For this review, take the finished solid that the model builds, in its own axes (mm). Face numbers are marked on the shaded views. Give positions to 0.01 mm unless a question says otherwise; leave off trailing zeros. Write each loop counter-clockwise with the first axis right and the second up, starting at its lowest first coordinate (ties: lowest second). Pieces come first, ordered by that corner, then holes.
1) We need section D-D on x = -21.5. Give the boundary of the cut face in (y, z), and give its area (3 significant figures).
2) For P1, Ø2, axis at x = -15, z = 26.5, coming from the +Y side; P2, Ø12, axis at x = -3, z = 56.5, coming from the -Y side; P3, Ø3.5, axis at y = -11.5, z = 37.5, coming from the +X side, all flat-tipped, find the tip position at first contact; note any pin that passes through.
3) We need section A-A on y = 0. Give the boundary of the cut face in (x, z), and give its area (3 significant figures).
4) We need section C-C on z = 46. Give the boundary of the cut face in (x, y).
5) Wall thickness on line 1 along Y through (x, z) = (10.75, 0.95); line 2 along Y through (x, z) = (3.5, 58); line 3 along Y through (x, z) = (-13.55, 21): over which ranges is each line inside the solid? List them lowest first.
6) We need section B-B on x = 0. Give the boundary of the cut face in (y, z), and give its area (3 significant figures).
7) Draft analysis for pull direction Y (two halves, no side actions). For the marked faces 1, 2 and 3, state which applies: pulls with the +Y half, pulls with the -Y half, needs draft (parallel to the pull), parting line crosses it, or undercut.
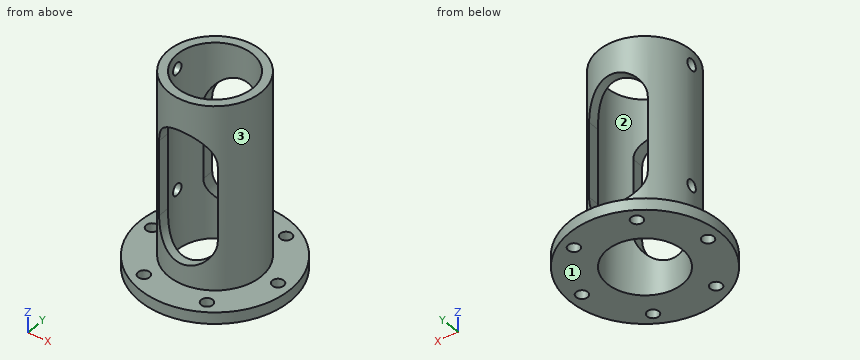
from build123d import *

# Parameters (mm, degrees)
SKETCH1_R           = 26
SKETCH1_R_2         = 13
SKETCH1_R_3         = 2
BOSS_EXTRUDE1_DEPTH = 4
SKETCH2_R           = 16
SKETCH2_R_2         = 13
BOSS_EXTRUDE2_DEPTH = 64
CUT_EXTRUDE1_DEPTH  = 32
SKETCH4_R           = 2
CUT_EXTRUDE2_DEPTH  = 64


with BuildPart() as part:
    # Sketch1 → Boss-Extrude1 (new body)
    with BuildSketch(Plane.XY):
        Circle(SKETCH1_R)
        Circle(SKETCH1_R_2, mode=Mode.SUBTRACT)
        with Locations((-21.5, 0)):
            Circle(SKETCH1_R_3, mode=Mode.SUBTRACT)
        with Locations((-10.75, 18.619546181)):
            Circle(SKETCH1_R_3, mode=Mode.SUBTRACT)
        with Locations((10.75, 18.619546181)):
            Circle(SKETCH1_R_3, mode=Mode.SUBTRACT)
        with Locations((21.5, 0)):
            Circle(SKETCH1_R_3, mode=Mode.SUBTRACT)
        with Locations((10.75, -18.619546181)):
            Circle(SKETCH1_R_3, mode=Mode.SUBTRACT)
        with Locations((-10.75, -18.619546181)):
            Circle(SKETCH1_R_3, mode=Mode.SUBTRACT)
    extrude(amount=BOSS_EXTRUDE1_DEPTH)

    # Sketch2 → Boss-Extrude2 (add)
    with BuildSketch(Plane.XY.offset(4)):
        Circle(SKETCH2_R)
        Circle(SKETCH2_R_2, mode=Mode.SUBTRACT)
    extrude(amount=BOSS_EXTRUDE2_DEPTH)

    # Sketch3 → Cut-Extrude1 (cut, symmetric)
    with BuildSketch(Plane(origin=(0, 0, 0), x_dir=(1, 0, 0), z_dir=(0, 1, 0))):
        with BuildLine():
            Line((10, -21), (10, -47))
            ThreePointArc((10, -47), (0, -57), (-10, -47))
            Line((-10, -47), (-10, -21))
            ThreePointArc((-10, -21), (0, -11), (10, -21))
        make_face()
    extrude(amount=CUT_EXTRUDE1_DEPTH, both=True, mode=Mode.SUBTRACT)

    # Sketch4 → Cut-Extrude2 (cut)
    with BuildSketch(Plane(origin=(0, 0, 0), x_dir=(0, 0, -1), z_dir=(1, 0, 0))):
        with Locations(Location((-21, 0, 0), (0, 0, 180))):
            Circle(SKETCH4_R)
        with Locations(Location((-63, 0, 0), (0, 0, 180))):
            Circle(SKETCH4_R)
    extrude(amount=-CUT_EXTRUDE2_DEPTH, mode=Mode.SUBTRACT)


solid = part.part
Results list:
1. outline: (-14.62, 0) - (-2, 0) - (-2, 4) - (-14.62, 4) - close; (2, 0) - (14.62, 0) - (14.62, 4) - (2, 4) - close
1. area: 101 mm2
2. P1: stops at y = 7.75
2. P2: stops at y = -16
2. P3: stops at x = 12.69
3. outline: (-26, 0) - (-23.5, 0) - (-23.5, 4) - (-26, 4) - close; (-19.5, 0) - (-13, 0) - (-13, 19) - (-16, 19) - (-16, 4) - (-19.5, 4) - close; (-16, 23) - (-13, 23) - (-13, 61) - (-16, 61) - close; (-16, 65) - (-13, 65) - (-13, 68) - (-16, 68) - close; (13, 0) - (19.5, 0) - (19.5, 4) - (16, 4) - (16, 68) - (13, 68) - close; (23.5, 0) - (26, 0) - (26, 4) - (23.5, 4) - close
3. area: 432 mm2
4. outline: (-10, -12.49) - (-10, -8.31) arc R13 cw to (-10, 8.31) - (-10, 12.49) arc R16 ccw to start; (10, -12.49) arc R16 ccw to (10, 12.49) - (10, 8.31) arc R13 cw to (10, -8.31) - close
5. line 1: y = -23.67 to -20.62, -16.62 to -7.31, 7.31 to 16.62, 20.62 to 23.67
5. line 2: y = -15.61 to -12.52, 12.52 to 15.61
5. line 3: y = -8.51 to -2, 2 to 8.51
6. outline: (-26, 0) - (-13, 0) - (-13, 11) - (-16, 11) - (-16, 4) - (-26, 4) - close; (-16, 57) - (-13, 57) - (-13, 68) - (-16, 68) - close; (13, 0) - (26, 0) - (26, 4) - (16, 4) - (16, 11) - (13, 11) - close; (13, 57) - (16, 57) - (16, 68) - (13, 68) - close
6. area: 212 mm2
7. face 1: needs draft
7. face 2: undercut
7. face 3: parting line crosses it
